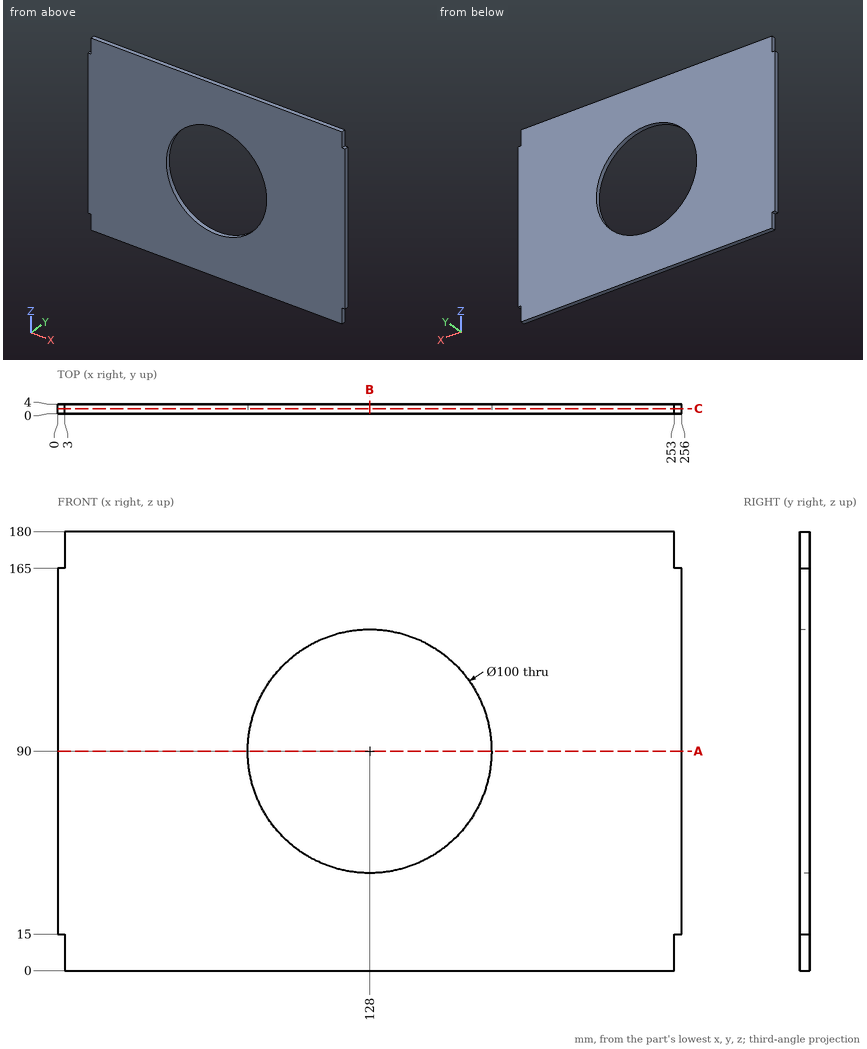
Geometry check sheet. Reference: drawing and pictorial views, mm from the part's lowest x, y, z. Round coordinates to 2 decimals unless told otherwise and drop trailing zeros. Order: outer loops, then holes, each group sorted by start corner. A loop starts at its lowest first (then second) coordinate and runs counter-clockwise, first axis right, second up. Notation, with made-up numbers: (48.5, 31.5) - (100.5, 31.5) arc R29 ccw to (100.5, 62.5) - close; hole circle Ø11 at (83, 36). An arc over 180 degrees is marked (long way). One line per question, with ' | ' between items. Start each with the question number.
(1) Depth check by flat-ended pin: pin 1 Ø1.2 at (y, z) = (2.5, 173.5) entering from +X; pin 2 Ø1.5 at (x, y) = (255, 2) entering from +Z; pin 3 Ø0.9 at (x, y) = (1.5, 2.5) entering from -Z. Enter the tip coordinate at first touch or a pass-through.
(2) Thickness scan on L1, parallel to X at y = 1.95, z = 90; L2, parallel to X at y = 0.55, z = 119.5; L3, parallel to Z at x = 154.5, y = 2.35. Record the ranges inside material, lowest first. Write a range as [from, to].
(3) Sectioned sample at A-A on z = 90. Record the cut outline in (x, y), and give its area (3 significant figures).
(4) Sectioned sample at B-B on x = 128. Record the cut outline in (y, z).
(5) Sectioned sample at C-C on y = 2.1. Record the cut outline in (x, z).
Conclusion:
1) pin 1: stops at x = 253 | pin 2: stops at z = 165 | pin 3: stops at z = 15
2) L1: x = [0, 78], [178, 256] | L2: x = [0, 87.63], [168.37, 256] | L3: z = [0, 47.6], [132.4, 180]
3) outline: (0, 0) - (78, 0) - (78, 4) - (0, 4) - close; (178, 0) - (256, 0) - (256, 4) - (178, 4) - close | area: 624 mm2
4) outline: (0, 0) - (4, 0) - (4, 40) - (0, 40) - close; (0, 140) - (4, 140) - (4, 180) - (0, 180) - close
5) outline: (0, 15) - (3, 15) - (3, 0) - (253, 0) - (253, 15) - (256, 15) - (256, 165) - (253, 165) - (253, 180) - (3, 180) - (3, 165) - (0, 165) - close; hole circle Ø100 at (128, 90)
